CAD build for the part. Positions are in the model's coordinates, mm. A direction names the side the tool comes from. Give positions to 0.01 mm unless a question says otherwise; leave off trailing zeros. Order: outer loops, then holes, each group sorted by start corner. A loop starts at its lowest first (then second) coordinate and runs counter-clockwise, first axis right, second up. Notation, with made-up numbers: (35, 58) -> (48, 58) arc R20 ccw to (48, 65) -> close; hole circle Ø8 at (-29.5, 83). An arc over 180 degrees is marked (long way). Answer as CSV lines item,"result".
```python
from build123d import *

# Parameters (mm, degrees)
F0_W     = 23
F0_H     = 62
F0_W_2   = 38
F1_DEPTH = 1
F2_DEPTH = 10
F3_R     = 5


# Not quite as in the source:
# - a feature names something its author has since deleted; it is built from what else it names


with BuildPart() as f1:
    # F0 (on Top) → F1 (new body)
    with BuildSketch(Plane.XY):
        with Locations((-21, 19)):
            Rectangle(F0_W, F0_H)
        with Locations((9.5, 19)):
            Rectangle(F0_W_2, F0_H)
        with BuildLine():
            ThreePointArc((9.5, 15.8775010008), (10.0985618966, 14.4432029131), (10.9121369044, 13.1189736826))
            Line((10.9121369044, 13.1189736826), (10.9121369044, 5.8810263174))
            ThreePointArc((10.9121369044, 5.8810263174), (10.0985618966, 4.5567970869), (9.5, 3.1224989992))
            ThreePointArc((9.5, 3.1224989992), (8.9014381034, 4.5567970869), (8.0878630956, 5.8810263174))
            Line((8.0878630956, 5.8810263174), (8.0878630956, 13.1189736826))
            ThreePointArc((8.0878630956, 13.1189736826), (8.9014381034, 14.4432029131), (9.5, 15.8775010008))
        make_face(mode=Mode.SUBTRACT)
        with BuildLine():
            Line((8.0878630956, 24.8810263174), (8.0878630956, 32.1189736826))
            ThreePointArc((8.0878630956, 32.1189736826), (8.9014381034, 33.4432029131), (9.5, 34.8775010008))
            ThreePointArc((9.5, 34.8775010008), (10.0985618966, 33.4432029131), (10.9121369044, 32.1189736826))
            Line((10.9121369044, 32.1189736826), (10.9121369044, 24.8810263174))
            ThreePointArc((10.9121369044, 24.8810263174), (10.0985618966, 23.5567970869), (9.5, 22.1224989992))
            ThreePointArc((9.5, 22.1224989992), (8.9014381034, 23.5567970869), (8.0878630956, 24.8810263174))
        make_face(mode=Mode.SUBTRACT)
    extrude(amount=F1_DEPTH)

    # F0 (on Top) → F2 (join)
    with BuildSketch(Plane.XY):
        with BuildLine():
            ThreePointArc((9.5, 34.8775010008), (8.9014381034, 33.4432029131), (8.0878630956, 32.1189736826))
            Line((8.0878630956, 32.1189736826), (8.0878630956, 24.8810263174))
            ThreePointArc((8.0878630956, 24.8810263174), (8.9014381034, 23.5567970869), (9.5, 22.1224989992))
            ThreePointArc((9.5, 22.1224989992), (10.0985618966, 23.5567970869), (10.9121369044, 24.8810263174))
            Line((10.9121369044, 24.8810263174), (10.9121369044, 32.1189736826))
            ThreePointArc((10.9121369044, 32.1189736826), (10.0985618966, 33.4432029131), (9.5, 34.8775010008))
        make_face()
        with BuildLine():
            Line((10.9121369044, 5.8810263174), (10.9121369044, 13.1189736826))
            ThreePointArc((10.9121369044, 13.1189736826), (10.0985618966, 14.4432029131), (9.5, 15.8775010008))
            ThreePointArc((9.5, 15.8775010008), (8.9014381034, 14.4432029131), (8.0878630956, 13.1189736826))
            Line((8.0878630956, 13.1189736826), (8.0878630956, 5.8810263174))
            ThreePointArc((8.0878630956, 5.8810263174), (8.9014381034, 4.5567970869), (9.5, 3.1224989992))
            ThreePointArc((9.5, 3.1224989992), (10.0985618966, 4.5567970869), (10.9121369044, 5.8810263174))
        make_face()
    extrude(amount=F2_DEPTH)

    # F3
    f3_edges = [f1.edges().sort_by_distance(p)[0] for p in [
        (-32.5, 50, 0.5),
        (28.5, 50, 0.5),
        (28.5, -12, 0.5),
        (-32.5, -12, 0.5),
    ]]
    fillet(f3_edges, radius=F3_R)


solid = f1.part
```
1) Band-saw the part on C-C, the plane x = 4. Write the cut outline in (y, z).
Data:
outline,"(-12, 0) -> (50, 0) -> (50, 1) -> (-12, 1) -> close"
2) Pull direction Y, two halves, no side cores. Call faces 6 (the cylindrical face through (8.89, 4.58, 5.44)), 7 (the cylindrical face through (8.91, 14.46, 5.44)), 8 (the flat face through (8.088, 10, 5)): pulls with the +Y half, pulls with the -Y half, needs draft (parallel to the pull), parting line crosses it, or undercut.
Data:
face 6,"pulls with the -Y half"
face 7,"undercut"
face 8,"needs draft"
3) Which spindle directions (+Z, -Z, +X, -X, +Y, -Y) get a long thin tool onto all of the face, cutting with end or side? Do faces 1 (the cylindrical face through (10.11, 33.42, 5.44)), 2 (the cylindrical face through (10.09, 23.54, 5.44)), 3 (the flat face through (8.088, 29, 5)), 4 (the flat face through (10.912, 9, 5)), 5 (the cylindrical face through (10.09, 4.54, 5.44)). Say none if no direction does.
Data:
face 1,"+Z, +X, +Y"
face 2,"+Z, +X"
face 3,"+Z, -X, +Y, -Y"
face 4,"+Z, +X, +Y, -Y"
face 5,"+Z, +X, -Y"
4) Band-saw the part on B-B, the plane y = 34. Write the cut outline in (x, z), then the cut area to 3 significant figures.
Data:
outline,"(-32.5, 0) -> (28.5, 0) -> (28.5, 1) -> (9.83, 1) -> (9.83, 10) -> (9.17, 10) -> (9.17, 1) -> (-32.5, 1) -> close"
area,"67.0 mm2"
5) Band-saw the part on D-D, the plane y = 41.5. Write the cut outline in (x, z).
Data:
outline,"(-32.5, 0) -> (28.5, 0) -> (28.5, 1) -> (-32.5, 1) -> close"
6) Band-saw the part on A-A, the plane z = 8. Write the cut outline in (x, y), then the cut area to 3 significant figures.
Data:
outline,"(8.09, 5.88) arc R10 cw to (9.5, 3.12) arc R10 cw to (10.91, 5.88) -> (10.91, 13.12) arc R10 cw to (9.5, 15.88) arc R10 cw to (8.09, 13.12) -> close; (8.09, 24.88) arc R10 cw to (9.5, 22.12) arc R10 cw to (10.91, 24.88) -> (10.91, 32.12) arc R10 cw to (9.5, 34.88) arc R10 cw to (8.09, 32.12) -> close"
area,"54.5 mm2"
7) Wall check: line 1 along Z through (x, y) = (-8.5, -2.5); line 2 along X through (y, z) = (27, 1.25); line 3 along X through (y, z) = (5.5, 9.5). Give the ranges that are in metal, low to high. Write a range as [from, to].
Data:
line 1,"z = [0, 1]"
line 2,"x = [8.09, 10.91]"
line 3,"x = [8.35, 10.65]"
8) Pin check, flat tips, straight feed: P1, Ø6, axis at y = 7.5, z = 7, coming from the +X side; P2, Ø6, axis at y = 27.5, z = 5, coming from the -X side; P3, Ø1.5, axis at x = 15, y = 36, coming from the +Z side. Stop position of each tip, or through.
Data:
P1,"stops at x = 10.91"
P2,"stops at x = 8.09"
P3,"stops at z = 1"
